```python
from build123d import *

# Parameters (mm, degrees)
SKETCH1_W           = 131
SKETCH1_H           = 89
BOSS_EXTRUDE1_DEPTH = 10
CUT_EXTRUDE1_DEPTH  = 100


with BuildPart() as part:
    # Sketch1 → Boss-Extrude1 (new body)
    with BuildSketch(Plane(origin=(0, 0, 0), x_dir=(1, 0, 0), z_dir=(0, 1, 0))):
        Rectangle(SKETCH1_W, SKETCH1_H)
    extrude(amount=BOSS_EXTRUDE1_DEPTH)

    # Sketch2 → Cut-Extrude1 (cut)
    # profile 1 of 2: a face of its own
    with BuildSketch(Plane(origin=(0, 10, 0), x_dir=(1, 0, 0), z_dir=(0, 1, 0))):
        Polygon((-62.5, 41.5), (-62.5, -41.5), (62.5, -41.5), (62.5, 36.324264069), (57.324264069, 41.5), align=None)
        Polygon((62.2, -41.2), (62.2, 36.2), (57.2, 41.2), (-62.2, 41.2), (-62.2, -41.2), align=None, mode=Mode.SUBTRACT)
    # profile 2 of 2: a face of its own
    with BuildSketch(Plane(origin=(0, 10, 0), x_dir=(1, 0, 0), z_dir=(0, 1, 0))):
        Polygon((-62.2, -41.2), (62.2, -41.2), (62.2, 36.2), (57.2, 41.2), (-62.2, 41.2), align=None)
    extrude(amount=-CUT_EXTRUDE1_DEPTH, mode=Mode.SUBTRACT)


solid = part.part
```
Geometry: final body of the model. Coordinates: model frame, mm. A direction names the side the tool comes from. Round coordinates to 2 decimals unless told otherwise and drop trailing zeros. Write each loop counter-clockwise with the first axis right and the second up, starting at its lowest first coordinate (ties: lowest second). Pieces come first, ordered by that corner, then holes.
Item 1: Section query B-B (x = -27.5). Return loops of the section in (y, z), plus the area to 3 significant figures.
Item 2: Section query C-C (y = 5). Return loops of the section in (x, z).
Item 3: Material intervals for L1, parallel to X at y = 9.25, z = 33; L2, parallel to Z at x = -6.5, y = 6; L3, parallel to Z at x = 58, y = 7.5, sorted ascending.
Item 4: Set-up query: faces 1 (the face through (65.5, 5, 1)), 2 (the face through (-1, 5, 41.5)). Return all of +Z, -Z, +X, -X, +Y, -Y with unobstructed straight access to the full face (end or side cutting, diameter ignored); none if empty.
Item 5: Mould query, pull axis Z, two halves, no side actions, for faces 3 (the face through (-1, 5, -44.5)), 4 (the face through (62.5, 5, 3)), 5 (the face through (-5, 0, 43)). Classes: +Z half, -Z half, draft (parallel to the pull), parting line (faces both ways), or undercut.
Item 6: Section query A-A (z = 0). Return loops of the section in (x, y).
Completed:
1. outline: (0, -44.5) - (10, -44.5) - (10, -41.5) - (0, -41.5) - close; (0, 41.5) - (10, 41.5) - (10, 44.5) - (0, 44.5) - close
1. area: 60.0 mm2
2. outline: (-65.5, -44.5) - (65.5, -44.5) - (65.5, 44.5) - (-65.5, 44.5) - close; hole (-62.5, -41.5) - (57.32, -41.5) - (62.5, -36.32) - (62.5, 41.5) - (-62.5, 41.5) - close
3. L1: x = -65.5 to -62.5, 62.5 to 65.5
3. L2: z = -44.5 to -41.5, 41.5 to 44.5
3. L3: z = -44.5 to -40.82, 41.5 to 44.5
4. face 1: +Z, -Z, +X, +Y, -Y
4. face 2: +Y, -Y
5. face 3: -Z half
5. face 4: undercut
5. face 5: draft
6. outline: (-65.5, 0) - (-62.5, 0) - (-62.5, 10) - (-65.5, 10) - close; (62.5, 0) - (65.5, 0) - (65.5, 10) - (62.5, 10) - close
